from build123d import *

# Parameters (mm, degrees)
F1_DEPTH = 8
F3_D     = 2.5
F5_D     = 2.5
F7_D     = 2.5
F8_F1_R  = 2.5
F8_F2_R  = 2.5
F9_D     = 2.5


with BuildPart() as f1:
    # F0 (on Top) → F1 (new body)
    with BuildSketch(Plane.XY):
        Polygon((-22.5, 35), (-30, 35), (-45.3108891325, 8.4807621135), (-15.3108891325, -43.4807621135), (15.3108891325, -43.4807621135), (45.3108891325, 8.4807621135), (30, 35), (22.5, 35), (22.5, 17.5), (22.5, -17.5), (-22.5, -17.5), (-22.5, 17.5), align=None)
        Polygon((-15.3108891325, -43.4807621135), (-45.3108891325, 8.4807621135), (-53.9711431703, 3.4807621135), (-23.9711431703, -48.4807621135), align=None)
        Polygon((30, 45), (-30, 45), (-30, 35), (-22.5, 35), (-22.5, 37.5), (22.5, 37.5), (22.5, 35), (30, 35), align=None)
        Polygon((53.9711431703, 3.4807621135), (45.3108891325, 8.4807621135), (15.3108891325, -43.4807621135), (23.9711431703, -48.4807621135), align=None)
    extrude(amount=F1_DEPTH)

    # F3 (through all)
    with Locations(Plane(origin=(-30, 0, 0), x_dir=(0, -1, 0), z_dir=(-1, 0, 0))):
        with Locations((-40, 4)):
            Hole(F3_D / 2)

    # F5 (through all)
    with Locations(Plane(origin=(15, -25.9807621135, 0), x_dir=(0.8660254038, 0.5, 0), z_dir=(0.5, -0.8660254038, 0))):
        with Locations((-40, 4)):
            Hole(F5_D / 2)

    # F7 (through all)
    with Locations(Plane(origin=(15, 25.9807621135, 0), x_dir=(-0.8660254038, 0.5, 0), z_dir=(0.5, 0.8660254038, 0))):
        with Locations((-40, 4)):
            Hole(F7_D / 2)

    # F8: fillet of radius 2.5 on 32 edges, made by hand

    # F8_f1
    f8_f1_edges = [f1.edges().sort_by_distance(p)[0] for p in [
        (-45.3108891325, 8.4807621135, 4),
        (-30, 35, 4),
        (30, 35, 4),
        (45.3108891325, 8.4807621135, 4),
        (15.3108891325, -43.4807621135, 4),
        (-15.3108891325, -43.4807621135, 4),
    ]]
    fillet(f8_f1_edges, radius=F8_F1_R)

    # F8_f2
    f8_f2_edges = [f1.edges().sort_by_distance(p)[0] for p in [
        (-37.6554445662, 21.7403810568, 8),
        (-30, 40.3349364905, 8),
        (0, 45, 8),
        (37.6554445662, 21.7403810568, 8),
        (30, 40.3349364905, 8),
        (49.9310796608, 5.8132938683, 8),
        (38.9711431703, -22.5, 8),
        (19.9310796608, -46.1482303588, 8),
        (0, -43.4807621135, 8),
        (-19.9310796608, -46.1482303588, 8),
        (-38.9711431703, -22.5, 8),
        (-49.9310796608, 5.8132938683, 8),
        (-53.9711431703, 3.4807621135, 4),
        (-30, 45, 4),
        (30, 45, 4),
        (53.9711431703, 3.4807621135, 4),
        (23.9711431703, -48.4807621135, 4),
        (-23.9711431703, -48.4807621135, 4),
        (-38.9711431703, -22.5, 0),
        (-37.6554445662, 21.7403810568, 0),
        (0, 45, 0),
        (30, 40.3349364905, 0),
        (38.9711431703, -22.5, 0),
        (19.9310796608, -46.1482303588, 0),
        (0, -43.4807621135, 0),
        (-19.9310796608, -46.1482303588, 0),
        (-15.2880637641, -43.5659475478, 0),
        (15.2880637641, -43.5659475478, 0),
        (30.0851854343, 35.0228253683, 0),
        (-30.0851854343, 35.0228253683, 0),
        (-45.3732491984, 8.5431221795, 0),
        (-45.3732491984, 8.5431221795, 8),
        (-15.2880637641, -43.5659475478, 8),
        (15.2880637641, -43.5659475478, 8),
        (45.3732491984, 8.5431221795, 8),
        (30.0851854343, 35.0228253683, 8),
        (-30.0851854343, 35.0228253683, 8),
    ]]
    fillet(f8_f2_edges, radius=F8_F2_R)

    # F9 (through all)
    with Locations(Plane(origin=(0, 0, 0), x_dir=(1, 0, 0), z_dir=(0, 0, -1))):
        with Locations((-27, -6.5), (-27, 9.5), (27, 9.5), (27, -6.5), (-27, -34.5), (27, -34.5)):
            Hole(F9_D / 2)


solid = f1.part
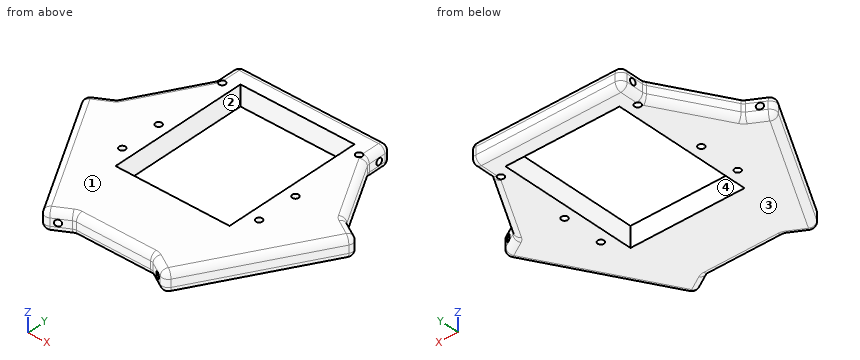
Could you check a few things on this model? Use its own coordinates, in mm. Face numbers are marked on the shaded views. A direction names the side the tool comes from. Round coordinates to 2 decimals unless told otherwise and drop trailing zeros. Order: outer loops, then holes, each group sorted by start corner. A loop starts at its lowest first (then second) coordinate and runs counter-clockwise, first axis right, second up.
Q1. I'm going to push flat-ended pins straight in: P1, Ø2, axis at y = -17.5, z = 3, coming from the +X side; P2, Ø3, axis at y = 10.5, z = 3, coming from the -X side; P3, Ø4, axis at y = 8.5, z = 4.5, coming from the +X side. Where does each tip first touch, or does it pass through?
Geometry says:
P1: stops at x = 42.44
P2: stops at x = -45.01
P3: stops at x = 48.73
Q2. Imagine slicing it at B-B, the plane z = 4. State how many separate pieces and enclosed holes the cut face has, then the cut area to 3 significant figures.
Geometry says:
separate pieces: 4
enclosed holes: 7
area: 3,980 mm2
Q3. Thinking about a two-plate mould opening in X: for the marked faces 1 and 2, which applies, released by +X, released by -X, zero draft, split by the parting line, or undercut?
Geometry says:
face 1: zero draft
face 2: undercut
Q4. Imagine slicing it at A-A, the plane x = -5. List the corners of the cut face in (y, z) for me.
Geometry says:
outline: (-43.48, 2.5) arc R2.5 ccw to (-40.98, 0) - (-17.5, 0) - (-17.5, 8) - (-40.98, 8) arc R2.5 ccw to (-43.48, 5.5) - close; (37.5, 0) - (42.5, 0) arc R2.5 ccw to (45, 2.5) - (45, 5.5) arc R2.5 ccw to (42.5, 8) - (37.5, 8) - close; hole circle Ø2.5 at (40, 4)
Q5. Which directions (+Z, -Z, +X, -X, +Y, -Y) give clear straight access to the entire face, cutting with the end or side of a thin tool? Please do the marked faces 3 and 4.
Geometry says:
face 3: -Z, +X, -X, +Y, -Y
face 4: +Z, -Z
Q6. Please list where these lines run through material, in increasing order: probe 1 along Y at (x, z) = (10, 3.75); probe 2 along Y at (x, z) = (-27, 6.5); probe 3 along X at (y, z) = (-9.5, 2.5).
Geometry says:
probe 1: y = -43.48 to -17.5, 37.5 to 38.78, 41.22 to 45
probe 2: y = -42.82 to -10.75, -8.25 to 5.25, 7.75 to 33.25, 35.75 to 44.79
probe 3: x = -46.48 to -28.25, -25.75 to -22.5, 22.5 to 25.75, 28.25 to 46.48
